Geometry check sheet. Reference: drawing and pictorial views, mm from the part's lowest x, y, z. Give positions to 0.01 mm unless a question says otherwise; leave off trailing zeros. Order: outer loops, then holes, each group sorted by start corner. A loop starts at its lowest first (then second) coordinate and runs counter-clockwise, first axis right, second up. Notation, with made-up numbers: (19, -5) -> (45, -5) arc R26 ccw to (45, 31) -> close; hole circle Ø1 at (43.5, 32.25). An arc over 180 degrees is marked (long way). Write each question's results on one line, items separated by ' | '.
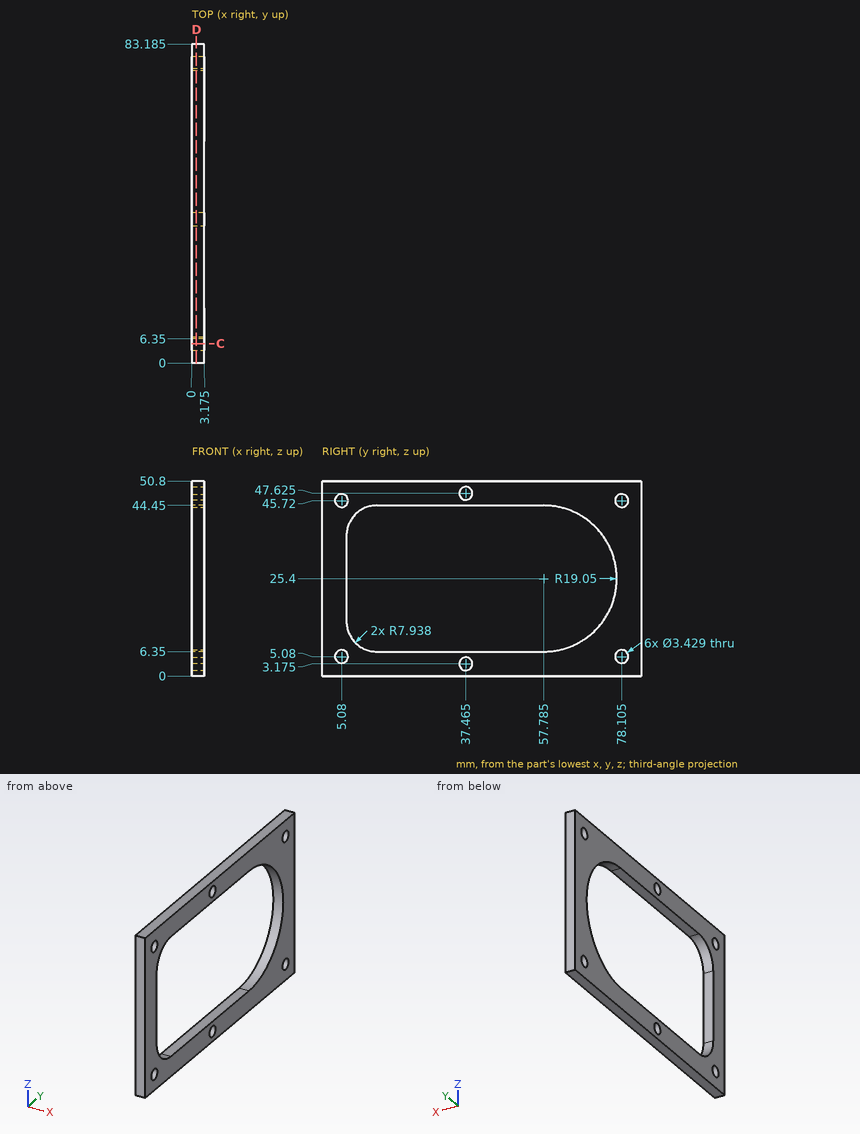
1. Gauge pin test, flat ends, axial feed: pin 1 Ø4 at (y, z) = (78.105, 45.72) entering from +X (1 decimal); pin 2 Ø2 at (y, z) = (5.08, 5.08) entering from +X. Record the tip position at first contact, or that the pin passes through.
Verdict:
pin 1: stops at x = 3.2 | pin 2: passes through
2. Material ranges on probe 1 along Z at (x, y) = (2.5, 5); probe 2 along Z at (x, y) = (2.8, 27.5); probe 3 along Y at (x, z) = (3, 5) (1 decimal), recorded low to high. Write a range as from..to.
Verdict:
probe 1: z = 0..3.37, 6.79..44.01, 47.43..50.8 | probe 2: z = 0..6.35, 44.45..50.8 | probe 3: y = 0..3.4, 6.8..76.4, 79.8..83.2
3. Section check C-C on y = 5.08. Record the cut outline in (x, z) (1 decimal).
Verdict:
outline: (0, 0) -> (3.2, 0) -> (3.2, 3.4) -> (0, 3.4) -> close; (0, 6.8) -> (3.2, 6.8) -> (3.2, 44) -> (0, 44) -> close; (0, 47.4) -> (3.2, 47.4) -> (3.2, 50.8) -> (0, 50.8) -> close
4. Section check D-D on x = 1.2. Give the number of separate pieces and of enclosed holes in the cut face, then the cut area to 3 significant figures.
Verdict:
separate pieces: 1 | enclosed holes: 7 | area: 1,670 mm^2
